Could you check a few things on this model? Use its own coordinates, in mm. A direction names the side the tool comes from. Coordinates: 2 decimals unless noted, no trailing zeros. Write each loop counter-clockwise with the first axis right and the second up, starting at its lowest first coordinate (ties: lowest second). Pieces come first, ordered by that corner, then holes.
Item 1: If I drill on probe 1 along Z at (x, y) = (0, -101.5); probe 2 along Y at (x, z) = (0, 19); probe 3 along Y at (x, z) = (0, 10.5), over which ranges is the centre line in solid material (lowest first)?
Item 2: Which directions (+Z, -Z, +X, -X, +Y, -Y) give clear straight access to the entire face, cutting with the end or side of a thin tool? Please do faces 5 (the flat face through (0, -18, -17.5)), 6 (the flat face through (7, -10, 17.5)), 7 (the cylindrical face through (-14.985, -133.6, 0.66)).
Item 3: Thinking about a two-plate mould opening in Y: for faces 1 (the cylindrical face through (-1.302, -7.585, 19.472)), 2 (the cylindrical face through (-11.99, -133.6, 0.53)), 3 (the flat face through (0, 0, 0)), 4 (the cylindrical face through (-0.78, -11.55, 10.24)), which applies, +Y half, -Y half, draft (parallel to the pull), parting line (faces both ways), or undercut?
Item 4: I want a section at C-C on y = -159.5. Please give me the cut outline in (x, z).
Item 5: I want a section at A-A on z = 0. Please give me the cut outline in (x, y).
Item 6: I want a section at D-D on y = -17.5. Please give me the cut outline in (x, z), then the cut area to 3 significant figures.
Item 7: For P1, Ø1, axis at y = -39.5, z = -9, coming from the -X side; P2, Ø4, axis at y = -162, z = -6, coming from the +X side; P3, Ø12, axis at x = 0.5, z = 21.5, coming from the +Y side; P4, Ø6, axis at y = -130, z = 13, coming from the +X side, each with a flat end and sliding along its axis, tell me the tip position at first contact or that it passes through.
from build123d import *

# Parameters (mm, degrees)
F0_W      = 35
F0_H      = 35
F1_DEPTH  = 35
F2_R      = 15
F2_R_2    = 12
F3_DEPTH  = 200
F4_R      = 10
F5_DEPTH  = 5
F6_R      = 8
F7_DEPTH  = 5
F8_SIZE   = 1
F9_SIZE   = 0.5
F10_R     = 6
F11_DEPTH = 35
F12_SIZE  = 0.5


# Not quite as in the source:
# - a feature names something its author has since deleted; it is built from what else it names


with BuildPart() as f1:
    # F0 (on Front) → F1 (new body)
    with BuildSketch(Plane.XZ):
        Rectangle(F0_W, F0_H)
    extrude(amount=F1_DEPTH)

    # F2 (on face) → F3 (join)
    with BuildSketch(Plane.XZ.offset(35)):
        Circle(F2_R)
        Circle(F2_R_2, mode=Mode.SUBTRACT)
    extrude(amount=F3_DEPTH)

    # F4 (on face) → F5 (join)
    with BuildSketch(Plane.XY.offset(17.5)):
        with Locations((0, -17.5)):
            Circle(F4_R)
    extrude(amount=F5_DEPTH)

    # F6 (on face) → F7 (join)
    with BuildSketch(Plane.XY.offset(22.5)):
        with Locations((0, -17.5)):
            Circle(F6_R)
    extrude(amount=F7_DEPTH)

    # F8
    f8_edges = [f1.edges().sort_by_distance(p)[0] for p in [
        (-10, -17.5, 22.5),
    ]]
    chamfer(f8_edges, length=F8_SIZE)

    # F9
    f9_edges = [f1.edges().sort_by_distance(p)[0] for p in [
        (-8, -17.5, 27.5),
    ]]
    chamfer(f9_edges, length=F9_SIZE)

    # F10 (on face) → F11 (cut)
    with BuildSketch(Plane.XY.offset(27.5)):
        with Locations((0, -17.5)):
            Circle(F10_R)
    extrude(amount=-F11_DEPTH, mode=Mode.SUBTRACT)

    # F12
    f12_edges = [f1.edges().sort_by_distance(p)[0] for p in [
        (0, -35, 17.5),
        (-17.5, -17.5, 17.5),
        (17.5, -17.5, 17.5),
        (0, 0, 17.5),
        (17.5, 0, 0),
        (17.5, -35, 0),
        (17.5, -17.5, -17.5),
        (0, 0, -17.5),
        (-17.5, -35, 0),
        (-17.5, -17.5, -17.5),
        (-17.5, 0, 0),
    ]]
    chamfer(f12_edges, length=F12_SIZE)


solid = f1.part
Response values:
1. probe 1: z = -15 to -12, 12 to 15
1. probe 2: y = -27.5 to -23.5, -11.5 to -7.5
1. probe 3: y = -35 to -23.5, -11.5 to 0
2. face 5: -Z, +X, -X, +Y, -Y
2. face 6: +Z
2. face 7: -Y
3. face 1: parting line
3. face 2: draft
3. face 3: +Y half
3. face 4: undercut
4. outline: circle Ø30 at (0, 0); hole circle Ø24 at (0, 0)
5. outline: (-17.5, -34.5) - (-17, -35) - (-15, -35) - (-15, -235) - (-12, -235) - (-12, -35) - (12, -35) - (12, -235) - (15, -235) - (15, -35) - (17, -35) - (17.5, -34.5) - (17.5, -0.5) - (17, 0) - (-17, 0) - (-17.5, -0.5) - close; hole circle Ø12 at (0, -17.5)
6. outline: (-17.5, -17) - (-17, -17.5) - (17, -17.5) - (17.5, -17) - (17.5, 17) - (17, 17.5) - (10, 17.5) - (10, 21.5) - (9, 22.5) - (8, 22.5) - (8, 27) - (7.5, 27.5) - (6, 27.5) - (6, -7.5) - (-6, -7.5) - (-6, 27.5) - (-7.5, 27.5) - (-8, 27) - (-8, 22.5) - (-9, 22.5) - (-10, 21.5) - (-10, 17.5) - (-17, 17.5) - (-17.5, 17) - close
6. area: 983 mm2
7. P1: stops at x = -12.36
7. P2: stops at x = 14.46
7. P3: stops at y = 0
7. P4: stops at x = 11.18
